Part model, mm, in its own coordinate system. A direction names the side the tool comes from. Round coordinates to 2 decimals unless told otherwise and drop trailing zeros. Write each loop counter-clockwise with the first axis right and the second up, starting at its lowest first coordinate (ties: lowest second). Pieces come first, ordered by that corner, then holes.
1) Saw through at B-B on z = 3. Write the cut outline in (x, y) (3 decimals).
2) Saw through at C-C on x = 23.25. Write the cut outline in (y, z).
3) Saw through at D-D on z = 6.25. Write the cut outline in (x, y) (3 decimals), and give its area (3 significant figures).
4) Saw through at A-A on x = 3.5. Write the cut outline in (y, z).
5) Which spindle directions (+Z, -Z, +X, -X, +Y, -Y) get a long thin tool onto all of the face, cutting with end or side? Do faces 1 (the flat face through (-12, 20, 5)), 2 (the cylindrical face through (-16.5, -0.6, 2.2)), 3 (the cylindrical face through (7, 0, 5)). Say none if no direction does.
6) Drill centre lines: L1, parallel to X at y = 6.5, z = 5.75; L2, parallel to Y at x = -4.5, z = 5.65; L3, parallel to X at y = -9.5, z = 4.5. Where is each one in solid material? Low to high.
7) Pull direction Y, two halves, no side cores. Call faces 4 (the flat face through (-15, 25, 1)), 5 (the cylindrical face through (-3.58, -9.57, 5.48)): +Y half, -Y half, draft (parallel to the pull), parting line (faces both ways), or undercut.
8) Flat gauge pins, fed straight in: pin 1 (3 mm diameter, centred on x = -4.5, y = -7.79, fed in from +Z); pin 2 (3 mm diameter, centred on x = -7.5, z = 5, fed in from -Y); pin 3 (12 mm diameter, centred on x = 23.25, y = 0, fed in from -Z); pin 4 (1 mm diameter, centred on x = -9.5, z = 3, fed in from -Y). Where does each tip first touch, or does it go through?
```python
from build123d import *

# Parameters (mm, degrees)
CYLINDER008_R     = 2
CYLINDER008_DEPTH = 10
ARRAY002_COUNT    = 6
CYLINDER035_R     = 1
CYLINDER035_DEPTH = 10
CYLINDER009_R     = 2
CYLINDER009_DEPTH = 10
CYLINDER001_R     = 15
CYLINDER001_DEPTH = 4
CYLINDER_R        = 18
CYLINDER_DEPTH    = 7
CYLINDER002_R     = 5.25
CYLINDER002_DEPTH = 4
CYLINDER003_R     = 8.25
CYLINDER003_DEPTH = 6
ARRAY_COUNT       = 3


with BuildPart() as array002:
    # Cylinder008 → Cylinder008 (new body)
    with BuildSketch(Plane(origin=(9, 0, 0), x_dir=(1, 0, 0), z_dir=(0, 0, 1))):
        Circle(CYLINDER008_R)
    extrude(amount=CYLINDER008_DEPTH)

    # Array002: Array002 ×6 about axis
    array002_axis = Axis((0, 0, 0), (0, 0, 1))


with BuildPart() as array002_1:
    add(array002.part)
    for i in range(1, ARRAY002_COUNT):
        add(array002.part.rotate(array002_axis, i * 360 / ARRAY002_COUNT))


with BuildPart() as cylinder010:
    # Cylinder035 → Cylinder035 (new body)
    with BuildSketch(Plane(origin=(-13, 0, 3), x_dir=(0, 0, 1), z_dir=(-1, 0, 0))):
        Circle(CYLINDER035_R)
    extrude(amount=CYLINDER035_DEPTH)


with BuildPart() as fusion027:
    # Cylinder009 → Cylinder009 (new body)
    with BuildSketch(Plane.XY):
        Circle(CYLINDER009_R)
    extrude(amount=CYLINDER009_DEPTH)

    # Fusion027: union Array002, Cylinder010
    add(array002_1.part)
    add(cylinder010.part)


with BuildPart() as cylinder001:
    # Cylinder001 → Cylinder001 (new body)
    with BuildSketch(Plane.XY):
        Circle(CYLINDER001_R)
    extrude(amount=CYLINDER001_DEPTH)


with BuildPart() as cut:
    # Cylinder → Cylinder (new body)
    with BuildSketch(Plane.XY):
        Circle(CYLINDER_R)
    extrude(amount=CYLINDER_DEPTH)

    # Cut: cut Cylinder001
    add(cylinder001.part, mode=Mode.SUBTRACT)


with BuildPart() as cylinder002:
    # Cylinder002 → Cylinder002 (new body)
    with BuildSketch(Plane.XY):
        Circle(CYLINDER002_R)
    extrude(amount=CYLINDER002_DEPTH)


with BuildPart() as toplevelpart_materialtestholder:
    # Cylinder003 → Cylinder003 (new body)
    with BuildSketch(Plane.XY):
        Circle(CYLINDER003_R)
    extrude(amount=CYLINDER003_DEPTH)

    # Cut001: cut Cylinder002
    add(cylinder002.part, mode=Mode.SUBTRACT)


with BuildPart() as toplevelpart_materialtestholder_1:
    # Cut001 placement: moved
    add(toplevelpart_materialtestholder.part.moved(Location((23.25, 0, 1))))

    # Array: TopLevelPart-MaterialTestHolder ×3 about axis
    array_axis = Axis((0, 0, 0), (0, 0, 1))


with BuildPart() as toplevelpart_materialtestholder_2:
    add(toplevelpart_materialtestholder_1.part)
    for i in range(1, ARRAY_COUNT):
        add(toplevelpart_materialtestholder_1.part.rotate(array_axis, i * 360 / ARRAY_COUNT))

    # Fusion: union Cut
    add(cut.part)

    # Cut006: cut Fusion027
    add(fusion027.part, mode=Mode.SUBTRACT)


solid = toplevelpart_materialtestholder_2.part
```
Completed:
1. outline: (-17.972, -1) arc R18 ccw to (-13.355, -12.068) arc R8.25 ccw (long way) to (-3.774, -17.6) arc R18 ccw to (17.129, -5.531) arc R8.25 ccw (long way) to (17.129, 5.531) arc R18 ccw to (-3.774, 17.6) arc R8.25 ccw (long way) to (-13.355, 12.068) arc R18 ccw to (-17.972, 1) - (-14.967, 1) arc R15 cw (long way) to (-14.967, -1) - close; hole circle Ø10.5 at (-11.625, -20.135); hole circle Ø10.5 at (-11.625, 20.135); hole circle Ø10.5 at (23.25, 0)
2. outline: (-8.25, 1) - (-5.25, 1) - (-5.25, 5) - (5.25, 5) - (5.25, 1) - (8.25, 1) - (8.25, 7) - (-8.25, 7) - close
3. outline: (-13.355, -12.068) arc R8.25 ccw (long way) to (-3.774, -17.6) arc R18 ccw to (17.129, -5.531) arc R8.25 ccw (long way) to (17.129, 5.531) arc R18 ccw to (-3.774, 17.6) arc R8.25 ccw (long way) to (-13.355, 12.068) arc R18 ccw to start; hole circle Ø4 at (-9, 0); hole circle Ø4 at (-4.5, -7.794); hole circle Ø4 at (-4.5, 7.794); hole circle Ø4 at (0, 0); hole circle Ø4 at (4.5, -7.794); hole circle Ø4 at (4.5, 7.794); hole circle Ø4 at (9, 0)
3. area: 1,500 mm2
4. outline: (-17.66, 0) - (-14.59, 0) - (-14.59, 4) - (-9.53, 4) - (-9.53, 7) - (-17.66, 7) - close; (-6.06, 4) - (6.06, 4) - (6.06, 7) - (-6.06, 7) - close; (9.53, 4) - (14.59, 4) - (14.59, 0) - (17.66, 0) - (17.66, 7) - (9.53, 7) - close
5. face 1: -Z
5. face 2: -X
5. face 3: +Z, -Z
6. L1: x = -16.79 to -6.02, -2.98 to 2.98, 6.02 to 16.79, 18.17 to 28.33
6. L2: y = -24.29 to -9.79, -5.79 to 5.79, 9.79 to 24.29
6. L3: x = -15.29 to -5.54, -3.46 to 3.46, 5.54 to 15.29
7. face 4: draft
7. face 5: undercut
8. pin 1: passes through
8. pin 2: stops at y = -27.96
8. pin 3: stops at z = 0
8. pin 4: stops at y = -28.22
